For this review, take the finished solid that the model builds, in its own axes (mm). Face numbers are marked on the shaded views. A direction names the side the tool comes from. Coordinates: 2 decimals unless noted, no trailing zeros. Write each loop counter-clockwise with the first axis right and the second up, starting at its lowest first coordinate (ties: lowest second). Pieces come first, ordered by that corner, then holes.
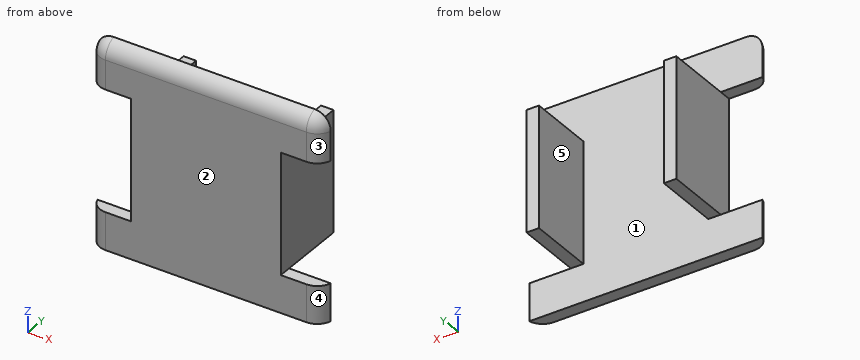
```python
from build123d import *

# Parameters (mm, degrees)
F1_DEPTH    = 12.271
F2_T1_DEPTH = 12.0635083269
F2_T4_ANGLE = 218.8024505591
F2_T6_ANGLE = 218.8024505591
F3_W        = 2.5
F3_H        = 7.2664258366
F4_DEPTH    = 0.751
F5_W        = 0.75
F5_H        = 7.2664258366
F6_DEPTH    = 4


# Not quite as in the source:
# - a fillet or chamfer that OpenCascade refuses, or shapes differently, is made with other operations: its cross-section is extruded or revolved along the edge and cut away or added


with BuildPart() as f1:
    # F0 (on Top) → F1 (new body)
    with BuildSketch(Plane.XY):
        with BuildLine():
            Line((1.5818497799, 3.6993569562), (-12.4181502201, 3.6993569562))
            ThreePointArc((-12.4181502201, 3.6993569562), (-12.0622768192, 3.1587875411), (-11.4499043835, 2.9493569562))
            Line((-11.4499043835, 2.9493569562), (0.6136039434, 2.9493569562))
            ThreePointArc((0.6136039434, 2.9493569562), (1.2259763791, 3.1587875411), (1.5818497799, 3.6993569562))
        make_face()
    extrude(amount=F1_DEPTH)

    # F2: fillet of radius 1 on 1 edges, made by hand

    # F2_s2 → F2_t1 (cut)
    with BuildSketch(Plane.YZ.offset(-11.4499043835)):
        with BuildLine():
            ThreePointArc((2.9493569562, 11.271), (3.242250175, 11.9781067812), (3.9493569562, 12.271))
            Line((3.9493569562, 12.271), (2.9493569562, 12.271))
            Line((2.9493569562, 12.271), (2.9493569562, 11.271))
        make_face()
    extrude(amount=F2_T1_DEPTH, mode=Mode.SUBTRACT)

    # F2_s3 → F2_t4 (revolve, cut)
    with BuildSketch(Plane(origin=(-8.8824733702, 7.1423174648, 0), x_dir=(0, 0, 1), z_dir=(0.7793111642, -0.6266371433, 0))):
        with BuildLine():
            ThreePointArc((11.271, 3.0971574071), (11.9781067812, 3.3900506259), (12.271, 4.0971574071))
            Line((12.271, 4.0971574071), (12.271, 3.0971574071))
            Line((12.271, 3.0971574071), (11.271, 3.0971574071))
        make_face()
    revolve(axis=Axis((-11.4499043835, 3.9493569562, 12.271), (0, 0, 1)), revolution_arc=F2_T4_ANGLE, mode=Mode.SUBTRACT)

    # F2_s5 → F2_t6 (revolve, cut)
    with BuildSketch(Plane.YZ.offset(0.6136039434)):
        with BuildLine():
            ThreePointArc((2.9493569562, 11.271), (3.242250175, 11.9781067812), (3.9493569562, 12.271))
            Line((3.9493569562, 12.271), (2.9493569562, 12.271))
            Line((2.9493569562, 12.271), (2.9493569562, 11.271))
        make_face()
    revolve(axis=Axis((0.6136039434, 3.9493569562, 12.271), (0, 0, 1)), revolution_arc=F2_T6_ANGLE, mode=Mode.SUBTRACT)

    # F3 (on face) → F4 (cut, through all)
    with BuildSketch(Plane(origin=(0, 3.6993569562, 0), x_dir=(-1, 0, 0), z_dir=(0, 1, 0))):
        with Locations((11.1681502201, 5.8831429183)):
            Rectangle(F3_W, F3_H)
        with Locations((-0.3318497799, 5.8831429183)):
            Rectangle(F3_W, F3_H)
    extrude(amount=-F4_DEPTH, mode=Mode.SUBTRACT)

    # F5 (on face) → F6 (join)
    with BuildSketch(Plane(origin=(0, 3.6993569562, 0), x_dir=(-1, 0, 0), z_dir=(0, 1, 0))):
        with Locations((1.2931502201, 5.8831429183)):
            Rectangle(F5_W, F5_H)
        with Locations((9.5431502201, 5.8831429183)):
            Rectangle(F5_W, F5_H)
    extrude(amount=F6_DEPTH)


solid = f1.part
```
Q1. For probe 1 along X at (y, z) = (5.7, 5.5); probe 2 along Y at (x, z) = (-5, 2.5); probe 3 along X at (y, z) = (3.35, 4), list the stretches that pass through material, from the lowest coordinate up.
Ans:
probe 1: x = -9.92 to -9.17, -1.67 to -0.92
probe 2: y = 2.95 to 3.7
probe 3: x = -9.92 to -0.92
Q2. Tool access review of the marked faces 4 and 5: name each direction out of +Z, -Z, +X, -X, +Y, -Y from which nothing blocks a thin tool from reaching the whole face with its end or side.
Ans:
face 4: +Z, -Z, +X, -Y
face 5: +Z, -Z, +Y
Q3. Add section B-B (y = 7.2). State the section outline as (x, z) points.
Ans:
outline: (-9.92, 2.25) - (-9.17, 2.25) - (-9.17, 9.52) - (-9.92, 9.52) - close; (-1.67, 2.25) - (-0.92, 2.25) - (-0.92, 9.52) - (-1.67, 9.52) - close
Q4. Add section A-A (x = -11.25). State the section outline as (y, z) points.
Ans:
outline: (2.95, 0) - (3.7, 0) - (3.7, 2.25) - (2.95, 2.25) - close; (2.95, 9.52) - (3.7, 9.52) - (3.7, 12.24) arc R1 ccw to (2.95, 11.27) - close
Q5. Add section D-D (x = -1.25). State the section outline as (y, z) points, then the cut area to 3 significant figures.
Ans:
outline: (2.95, 0) - (3.7, 0) - (3.7, 2.25) - (7.7, 2.25) - (7.7, 9.52) - (3.7, 9.52) - (3.7, 12.24) arc R1 ccw to (2.95, 11.27) - close
area: 38.1 mm2
Q6. Draft analysis for pull direction X (two halves, no side actions). For the marked faces 1, 2 and 3, state which applies: +X half, -X half, draft (parallel to the pull), parting line (faces both ways), or undercut.
Ans:
face 1: undercut
face 2: draft
face 3: +X half
Q7. Add section C-C (z = 6.5). State the section outline as (x, y) points, then the cut area to 4 significant figures.
Ans:
outline: (-9.92, 2.95) - (-0.92, 2.95) - (-0.92, 7.7) - (-1.67, 7.7) - (-1.67, 3.7) - (-9.17, 3.7) - (-9.17, 7.7) - (-9.92, 7.7) - close
area: 12.75 mm2
Q8. Clearance check with flat-ended pins moving along their axes: pin 1 Ø0.8 at (x, y) = (-9.5, 6.5) entering from -Z; pin 2 Ø0.8 at (x, y) = (-9.5, 5) entering from +Z; pin 3 Ø1.2 at (y, z) = (5, 7.5) entering from -X. State where each tip first meets the part, or that it passes through.
Ans:
pin 1: stops at z = 2.25
pin 2: stops at z = 9.52
pin 3: stops at x = -9.92
